Verification items for this drawing (mm, ordinates from the low corner). A direction names the side the tool comes from. Round coordinates to 2 decimals unless told otherwise and drop trailing zeros. Loops run counter-clockwise (first coordinate to the right, second up) from the corner with the lowest first, then second, coordinate; pieces in that order, holes last. Notation, with made-up numbers: M 86,68.5 L 100,68.5 A26 ccw 100,86.5 Z; hole C 76,-20 d7. An arc over 180 degrees is marked long. One line per item, written item: value.
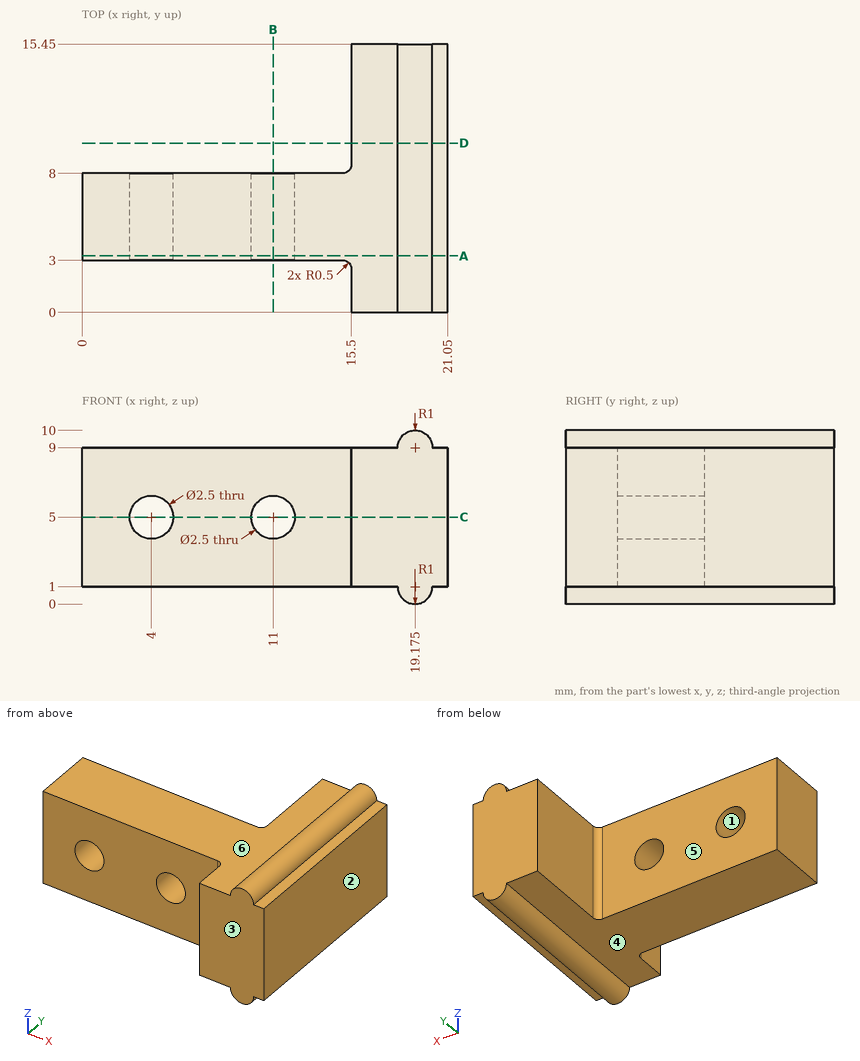
(1) Sectioned sample at A-A on y = 3.25. Enter the section's corners in (x, z) (3 decimals).
Completed:
outline: M 0,1 L 18.175,1 A1 ccw 20.175,1 L 21.05,1 L 21.05,9 L 20.175,9 A1 ccw 18.175,9 L 0,9 Z; hole C 4,5 d2.5; hole C 11,5 d2.5
(2) Tool access check on the marked faces 4, 5 and 6. Record the directions out of +Z, -Z, +X, -X, +Y, -Y that give a thin tool (end or side, any length) a straight path to the whole face; none if there is none.
Completed:
face 4: -Z, -X, +Y, -Y
face 5: +Z, -Z, -X, +Y
face 6: +Z, -X, +Y, -Y
(3) Thickness scan on L1, parallel to X at y = 5.2, z = 5; L2, parallel to X at y = 5.25, z = 4.25; L3, parallel to Z at x = 11, y = 7.75. Record the ranges inside material, lowest first. Write a range as from..to.
Completed:
L1: x = 0..2.75, 5.25..9.75, 12.25..21.05
L2: x = 0..3, 5..10, 12..21.05
L3: z = 1..3.75, 6.25..9
(4) Sectioned sample at C-C on z = 5. Enter the section's corners in (x, y).
Completed:
outline: M 0,3 L 2.75,3 L 2.75,8 L 0,8 Z; M 5.25,3 L 9.75,3 L 9.75,8 L 5.25,8 Z; M 12.25,3 L 15,3 A0.5 cw 15.5,2.5 L 15.5,0 L 21.05,0 L 21.05,15.45 L 15.5,15.45 L 15.5,8.5 A0.5 cw 15,8 L 12.25,8 Z
(5) Sectioned sample at B-B on x = 11. Enter the section's corners in (y, z).
Completed:
outline: M 3,1 L 8,1 L 8,3.75 L 3,3.75 Z; M 3,6.25 L 8,6.25 L 8,9 L 3,9 Z
(6) Mould release check, pull along X, two halves, no side actions. Record for the marked faces 1, 2 and 3: +X half, -X half, draft (parallel to the pull), parting line (faces both ways), or undercut.
Completed:
face 1: undercut
face 2: +X half
face 3: draft
(7) Depth check by flat-ended pin: pin 1 Ø3.5 at (y, z) = (10.5, 6.5) entering from -X; pin 2 Ø2.5 at (x, z) = (7.5, 6.5) entering from -Y; pin 3 Ø7.5 at (x, y) = (10, 8.5) entering from -Z. Enter the tip coordinate at first touch or a pass-through.
Completed:
pin 1: stops at x = 15.5
pin 2: stops at y = 3
pin 3: stops at z = 1
(8) Sectioned sample at D-D on y = 9.75. Enter the section's corners in (x, z) (3 decimals).
Completed:
outline: M 15.5,1 L 18.175,1 A1 ccw 20.175,1 L 21.05,1 L 21.05,9 L 20.175,9 A1 ccw 18.175,9 L 15.5,9 Z
